Read the model definition and answer for the solid it produces. Units are mm, in the model's axes. A direction names the side the tool comes from. Round coordinates to 2 decimals unless told otherwise and drop trailing zeros. Loops run counter-clockwise (first coordinate to the right, second up) from the corner with the lowest first, then second, coordinate; pieces in that order, holes last. Notation, with made-up numbers: (41, 19) - (91, 19) arc R15 cw to (91, 44) - close; hole circle Ø4 at (15, 49.25). An arc over 180 degrees is marked (long way). Use one line per item in the form item = value. Start each with the question number.
Autodesk Inventor part; units mm, degrees
ref_plane "YZ Plane" through (0, 0, 0) normal (1, 0, 0) x (0, 1, 0)
ref_plane "XZ Plane" through (0, 0, 0) normal (0, 1, 0) x (-1, 0, 0)
ref_plane "XY Plane" through (0, 0, 0) normal (0, 0, 1) x (1, 0, 0)
sketch "スケッチ1" plane through (0, 0, 0) normal (1, 0, 0) x (0, 1, 0)
  line L0 (1.7321, -3) -> (-1.7321, -3)
  line L1 (-1.7321, -3) -> (-3.4641, 0)
  line L2 (-3.4641, 0) -> (-1.7321, 3)
  line L3 (-1.7321, 3) -> (1.7321, 3)
  line L4 (1.7321, 3) -> (3.4641, 0)
  line L5 (3.4641, 0) -> (1.7321, -3)
  point P0 (0, 0)
  point P1 (0, 0)
  dimension "d0" = 6
extrude "押し出し1" add sketch "スケッチ1" along normal blind 40
sketch "スケッチ2" plane through (40, 0, 0) normal (1, 0, 0) x (0, 0, -1)
  circle A0 centre (0, 0) radius 1.5
  dimension "d3" = 3
extrude "押し出し2" add sketch "スケッチ2" along normal blind 8
thread "ねじ1"
sketch "スケッチ3" plane through (0, 0, 0) normal (-1, 0, 0) x (0, 0, 1)
  point P0 (0, 0)
  point P1 (0, 0)
hole "穴1" at (0, 0, 0) direction (1, 0, 0) diameter 2.459 depth 10 tip angle 118
properties part number "Spacer_M3_L15" material "鋼、合金"
1) A cutting plane is placed at A-A on x = 5.5. Write down the section's boundary in (y, z).
2) Determine the mould class of faces 4 (the conical face through (10.61, 0.064, 0.204)), 5 (the flat face through (19.7, -2.6, 1.5)), 6 (the cylindrical face through (43.94, -0.07, 1.5)) for opening direction Y: +Y half, -Y half, draft (parallel to the pull), parting line (faces both ways), or undercut.
3) A cutting plane is placed at B-B on x = 38. Write down the section's boundary in (y, z).
4) For faces 1 (the flat face through (48, 0, 0)), 2 (the cylindrical face through (5.07, 0.748, -0.976)), 3 (the flat face through (40, 1.5, 0.7)), determine the directions among +Z, -Z, +X, -X, +Y, -Y from which every point of the face is accessible in a straight line to the end or side of a thin tool.
5) Straight lines are drawn through the part: line 1 (Y direction, x = 3.75, z = 0); line 2 (Z direction, x = 5.75, y = 0); line 3 (X direction, y = 1, z = -1.55). For each, find the intervals that lie inside material, in ascending order. Write a range as from..to.
6) A cutting plane is placed at C-C on y = -2.25. Write down the section's boundary in (x, z).
7) A cutting plane is placed at D-D on z = 2.6. Write down the section's boundary in (x, y).
Checks:
q1.outline = (-3.46, 0) - (-1.73, -3) - (1.73, -3) - (3.46, 0) - (1.73, 3) - (-1.73, 3) - close; hole circle Ø2.46 at (0, 0)
q2.face_4 = undercut
q2.face_5 = -Y half
q2.face_6 = parting line
q3.outline = (-3.46, 0) - (-1.73, -3) - (1.73, -3) - (3.46, 0) - (1.73, 3) - (-1.73, 3) - close
q4.face_1 = +Z, -Z, +X, +Y, -Y
q4.face_2 = -X
q4.face_3 = +X
q5.line_1 = -3.46..-1.23, 1.23..3.46
q5.line_2 = -3..-1.23, 1.23..3
q5.line_3 = 0..40
q6.outline = (0, -2.1) - (40, -2.1) - (40, 2.1) - (0, 2.1) - close
q7.outline = (0, -1.96) - (40, -1.96) - (40, 1.96) - (0, 1.96) - close
